```python
from build123d import *

# Parameters (mm, degrees)
SKETCH_1_W      = 400
SKETCH_1_H      = 110
EXTRUDE_1_DEPTH = 125
FILLET_1_R      = 10
SHELL_1_T       = -3


with BuildPart() as part:
    # 草图1 → 凸台-拉伸1 (new body)
    with BuildSketch(Plane.XY):
        Rectangle(SKETCH_1_W, SKETCH_1_H)
    extrude(amount=EXTRUDE_1_DEPTH)

    # 圆角1
    fillet_1_edges = [part.edges().sort_by_distance(p)[0] for p in [
        (-200, 0, 125),
        (200, 0, 125),
        (0, 55, 125),
        (-200, 55, 62.5),
        (200, 55, 62.5),
    ]]
    fillet(fillet_1_edges, radius=FILLET_1_R)

    # 抽壳1
    shell_1_openings = [part.faces().sort_by_distance(p)[0] for p in [
        (0, 15.690355937, 0),
        (0, -55, 80.690355937),
    ]]
    offset(amount=SHELL_1_T, openings=shell_1_openings, kind=Kind.INTERSECTION)


solid = part.part
```
Can you work these out from the model? Positions are in its coordinate system, mm. A direction names the side the tool comes from. Coordinates: 2 decimals unless noted, no trailing zeros. Write each loop counter-clockwise with the first axis right and the second up, starting at its lowest first coordinate (ties: lowest second). Pieces come first, ordered by that corner, then holes. Notation, with made-up numbers: (60, 2) - (82, 2) arc R13 cw to (82, 16) - close; hole circle Ø6 at (49.25, -7.75). An arc over 180 degrees is marked (long way). Return JSON: item names as keys, results as strings.
Q1. If we section it at C-C (x = 104.5): Please give me the cut outline in (y, z).
Computed values:
{"outline": "(-55, 122) - (45, 122) arc R7 cw to (52, 115) - (52, 0) - (55, 0) - (55, 115) arc R10 ccw to (45, 125) - (-55, 125) - close"}
Q2. Thinking about a two-plate mould opening in X: for faces 3 (the cylindrical face through (-197.15, 51.99, 58.3)), 4 (the cylindrical face through (2.66, 52.15, 121.99)), 5 (the flat face through (-197, -6, 57)), which applies, +X half, -X half, draft (parallel to the pull), parting line (faces both ways), or undercut?
Computed values:
{"face 3": "-X half", "face 4": "draft", "face 5": "undercut"}
Q3. Please list where these lines run through material, in increasing order: L1, parallel to X at y = 8, z = 103; L2, parallel to Y at x = 64.5, z = 33; L3, parallel to Z at x = -67, y = -23. Write a range as from..to.
Computed values:
{"L1": "x = -200..-197, 197..200", "L2": "y = 52..55", "L3": "z = 122..125"}
Q4. On a 3-axis mill with a long thin cutter (end or side, diameter ignored), from which of +Z, -Z, +X, -X, +Y, -Y can I reach the whole of each face in a straight line? I mean faces 1 (the flat face through (-3, -4, 122)), 2 (the flat face through (-200, -6, 57)). Say none if no direction works.
Computed values:
{"face 1": "-Z, -Y", "face 2": "+Z, -Z, -X, +Y, -Y"}
Q5. If we section it at B-B (z = 8.5): Please give me the cut outline in (x, y).
Computed values:
{"outline": "(-200, -55) - (-197, -55) - (-197, 45) arc R7 cw to (-190, 52) - (190, 52) arc R7 cw to (197, 45) - (197, -55) - (200, -55) - (200, 45) arc R10 ccw to (190, 55) - (-190, 55) arc R10 ccw to (-200, 45) - close"}
Q6. If we section it at A-A (y = -21): Please give me the cut outline in (x, z).
Computed values:
{"outline": "(-200, 0) - (-197, 0) - (-197, 115) arc R7 cw to (-190, 122) - (190, 122) arc R7 cw to (197, 115) - (197, 0) - (200, 0) - (200, 115) arc R10 ccw to (190, 125) - (-190, 125) arc R10 ccw to (-200, 115) - close"}
